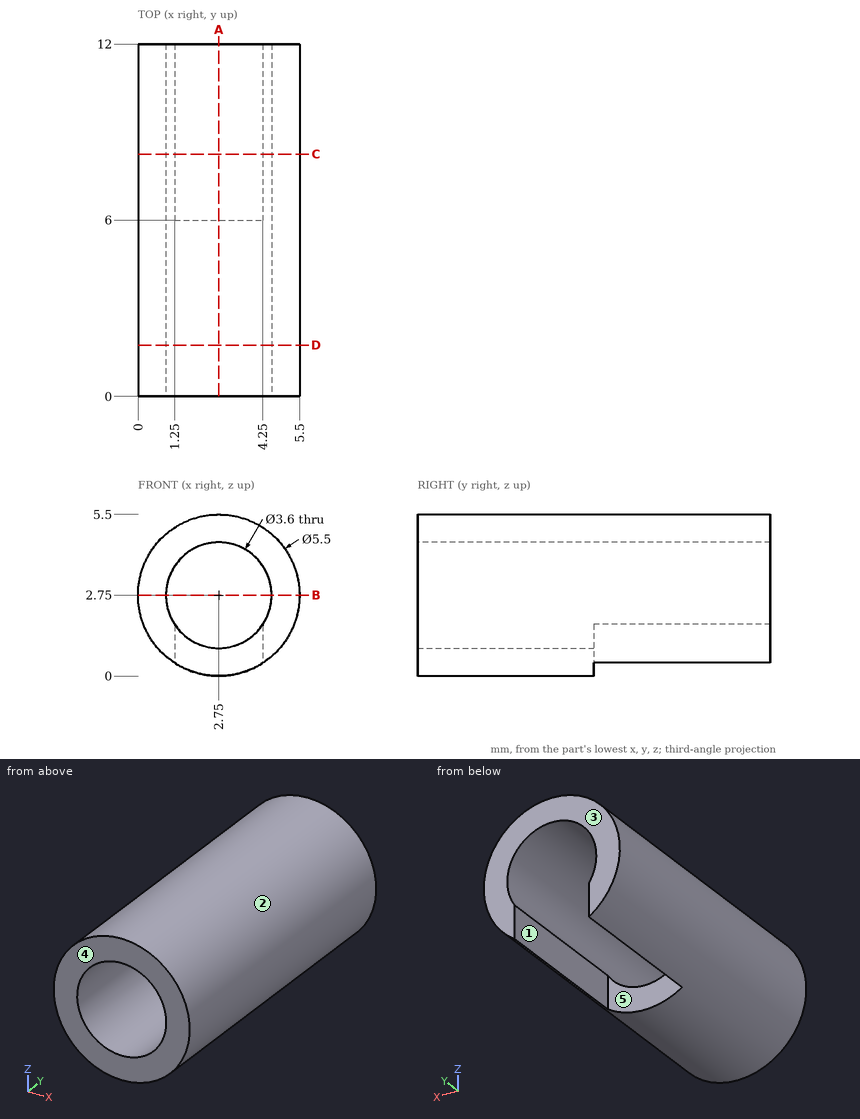
Answer from the drawing. Dimensions are ordinates in mm from the lowest x, y and z of the part. A direction names the side the tool comes from. Round coordinates to 2 decimals unless told otherwise and drop trailing zeros. Loops run counter-clockwise (first coordinate to the right, second up) from the corner with the lowest first, then second, coordinate; pieces in that order, holes last.
Q1. Section A-A on x = 2.75 is taken. Write down the section's boundary in (y, z), and give its area (3 significant figures).
Q2. Section D-D on y = 1.75 is taken. Write down the section's boundary in (x, z), and give its area (3 significant figures).
Q3. Determine the mould class of the marked faces 1, 2 and 3 for opening direction X: released by +X, released by -X, zero draft, split by the parting line, or undercut.
Q4. Each of these flat-tipped pins is pushed along its axis until it touches: pin 1 (1.5 mm diameter, centred on x = 4, y = 7, fed in from +Z); pin 2 (0.7 mm diameter, centred on y = 10, z = 1, fed in from -X); pin 3 (3 mm diameter, centred on x = 2.75, z = 2.75, fed in from +Y); pin 4 (0.9 mm diameter, centred on x = 3, z = 0.5, fed in from +Y). Where does it stop, or does it pass through?
Q5. Section B-B on z = 2.75 is taken. Write down the section's boundary in (x, y).
Q6. Which of the six approach directions +Z, -Z, +X, -X, +Y, -Y give full straight-line access (tool end or side, diameter ignored) to the marked faces 4 and 5?
Q7. Consider probe 1 along X at (y, z) = (4, 2.75); probe 2 along X at (y, z) = (4.25, 1.1); probe 3 along Z at (x, y) = (2.75, 7.75). Determine where each line is inside the solid, lowest interval first.
Q8. Section C-C on y = 8.25 is taken. Write down the section's boundary in (x, z).
Output:
1. outline: (0, 0) - (6, 0) - (6, 0.95) - (0, 0.95) - close; (0, 4.55) - (12, 4.55) - (12, 5.5) - (0, 5.5) - close
1. area: 17.1 mm2
2. outline: circle Ø5.5 at (2.75, 2.75); hole circle Ø3.6 at (2.75, 2.75)
2. area: 13.6 mm2
3. face 1: undercut
3. face 2: split by the parting line
3. face 3: zero draft
4. pin 1: stops at z = 5.45
4. pin 2: stops at x = 0.38
4. pin 3: passes through
4. pin 4: stops at y = 6
5. outline: (0, 0) - (0.95, 0) - (0.95, 12) - (0, 12) - close; (4.55, 0) - (5.5, 0) - (5.5, 12) - (4.55, 12) - close
6. face 4: +Z, -Z, +X, -X, -Y
6. face 5: -Z, +Y
7. probe 1: x = 0 to 0.95, 4.55 to 5.5
7. probe 2: x = 0.55 to 2.03, 3.47 to 4.95
7. probe 3: z = 4.55 to 5.5
8. outline: (1.25, 0.45) - (1.25, 1.76) arc R1.8 cw (long way) to (4.25, 1.76) - (4.25, 0.45) arc R2.75 ccw (long way) to start
